Job drawing, mm, ordinate dimensions from the low corner. One solid piece. Give positions to 0.01 mm unless a question says otherwise; leave off trailing zeros. Loops run counter-clockwise (first coordinate to the right, second up) from the corner with the lowest first, then second, coordinate; pieces in that order, holes last. Notation, with made-up numbers: (-19, 41.5) -> (19, 41.5) arc R20 cw to (19, 48.5) -> close; hole circle Ø11 at (11, 73). An arc over 180 degrees is marked (long way). Answer as a JSON object with one key per item and string values. Group by question number.
Q1. Band-saw the part on A-A, the plane z = 142. Write the cut outline in (x, y), plus the area to 3 significant figures.
Q2. Drop flat-ended pins along their axis: pin 1 (1.5 mm diameter, centred on x = 1.5, y = 1, fed in from -Z); pin 2 (1.5 mm diameter, centred on y = 2, z = 39.5, fed in from -X); pin 3 (0.9 mm diameter, centred on y = 1, z = 83, fed in from +X). Give the stop position or say it passes through.
Q3. Wall check: probe 1 along X at (y, z) = (1.7, 137.5); probe 2 along Z at (x, y) = (16.5, 2.6). Give the ranges that are in metal, low to high. Write a range as from..to.
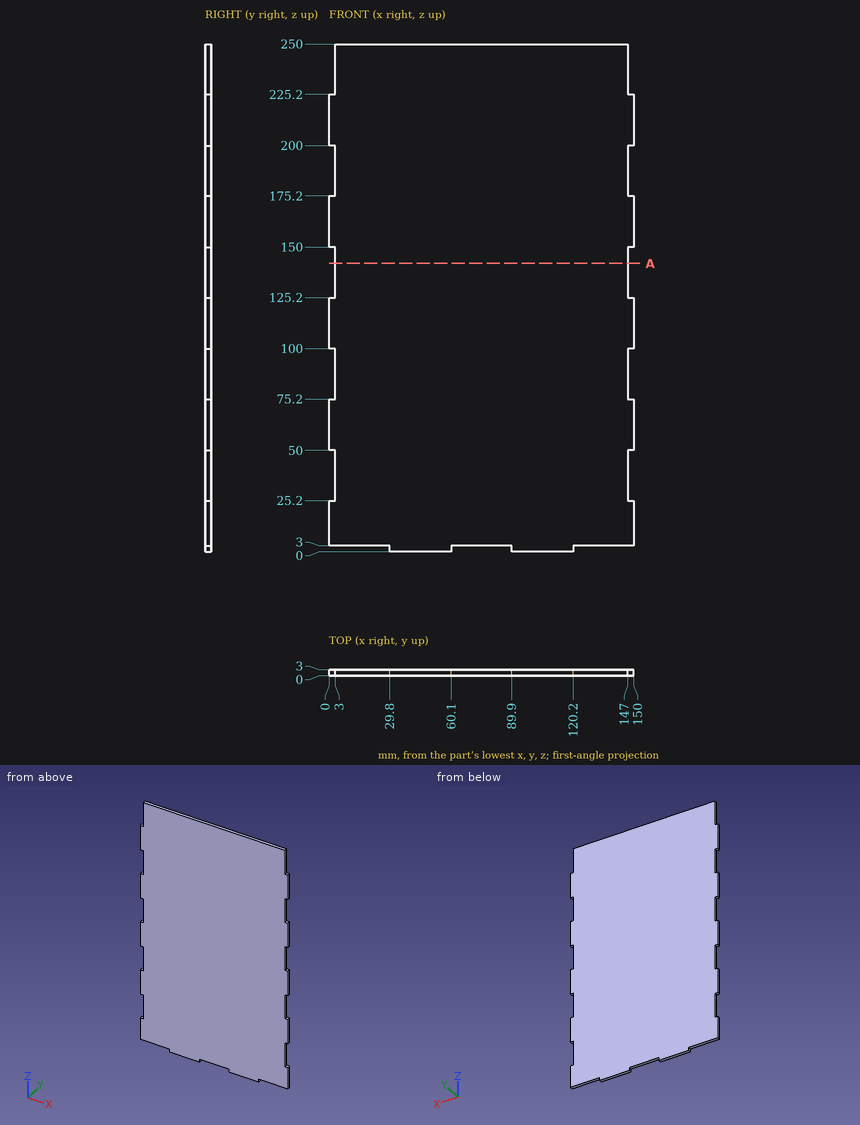
Worked answers:
{
 "1": {"outline": "(3, 0) -> (147, 0) -> (147, 3) -> (3, 3) -> close", "area": "432 mm2"},
 "2": {"pin 1": "z = 3", "pin 2": "x = 3", "pin 3": "x = 147"},
 "3": {"probe 1": "3..147", "probe 2": "3..250"}
}
